Build history of the part. All positions in model axes, mm. A direction names the side the tool comes from. Give positions to 0.01 mm unless a question says otherwise; leave off trailing zeros. Loops run counter-clockwise (first coordinate to the right, second up) from the corner with the lowest first, then second, coordinate; pieces in that order, holes last. Notation, with made-up numbers: (39.25, 15.5) -> (95.25, 15.5) arc R28 cw to (95.25, 46.5) -> close; hole circle Ø4 at (68, 40.5). An arc over 180 degrees is marked (long way). Answer as a JSON object with one key per item and string values. Group by question number.
from build123d import *

# Parameters (mm, degrees)
BOSS_EXTRUDE1_DEPTH = 3
BOSS_EXTRUDE2_DEPTH = 3


with BuildPart() as part:
    # Sketch1 → Boss-Extrude1 (new body)
    with BuildSketch(Plane.XY):
        Polygon((3, -5), (12.522083602, -5), (38.000000001, 65), (38.000000001, 70), (41, 70), (41, 89.999999997), (38.000000001, 89.999999997), (38.000000001, 94.999999997), (28.477916397, 94.999999997), (18.390906449, 67.286167933), (15.571828589, 68.312228362), (8.731425723, 49.518375949), (11.550503583, 48.49231552), (3, 25), (3, 20), (0, 20), (0, 0), (3, 0), align=None)
    extrude(amount=BOSS_EXTRUDE1_DEPTH)

    # Sketch2 → Boss-Extrude2 (add)
    with BuildSketch(Plane(origin=(0, 0, 0), x_dir=(-1, 0, 0), z_dir=(0, 0, -1))):
        Polygon((-7.955671859, 64.929836131), (-3.093269996, 51.57049681), (-8.731425723, 49.518375949), (-15.571828589, 68.312228362), (-18.390906449, 67.286167933), (-28.477916397, 94.999999997), (-18.900316445, 94.999999997), (-14.796074725, 83.723688547), (-11.976996863, 84.749748977), (-5.136593996, 65.955896561), align=None)
    extrude(amount=-BOSS_EXTRUDE2_DEPTH)


solid = part.part
(1) Saw through at C-C on y = 4.5. List the corners of the cut face in (x, z).
(2) Pin check, flat tips, straight feed: pin 1 (1.5 mm diameter, centred on y = 92, z = 1, fed in from +X); pin 2 (1.5 mm diameter, centred on y = 23, z = 1.5, fed in from -X). Stop position of each tip, or through.
(3) Pull direction Y, two halves, no side cores. Call faces 1 (the flat face through (5.559, 58.344, 1.479)), 2 (the flat face through (41, 80, 1)), 3 (the flat face through (13.41, 84.23, 1.48)): pulls with the +Y half, pulls with the -Y half, needs draft (parallel to the pull), parting line crosses it, or undercut.
(4) Saw through at A-A on z = 1. List the corners of the cut face in (x, y).
(5) 3-axis set-ups, long thin cutter, end or side, ignore diameter. For faces 4 (the flat face through (7.335, 36.911, 1.479)), 5 (the flat face through (3, 23, 1)), 6 (the flat face through (38, 92, 1)), 7 (the flat face through (38, 67, 1)): which of +Z, -Z, +X, -X, +Y, -Y reach the whole face in a straight line?
(6) Saw through at B-B on x = 17. List the corners of the cut face in (y, z), plus the area to 3 significant figures.
(7) Probe line 1 along Y through (x, z) = (2, 0.75); line 2 along Y through (x, z) = (12, 1); line 3 along X through (y, z) = (83, 2.15). List the from-to ranges inside material, lowest first. Write a range as [from, to].
Calculated:
{
 "1": {"outline": "(0, 0) -> (15.98, 0) -> (15.98, 3) -> (0, 3) -> close"},
 "2": {"pin 1": "stops at x = 38", "pin 2": "stops at x = 3"},
 "3": {"face 1": "undercut", "face 2": "needs draft", "face 3": "pulls with the +Y half"},
 "4": {"outline": "(0, 0) -> (3, 0) -> (3, -5) -> (12.52, -5) -> (38, 65) -> (38, 70) -> (41, 70) -> (41, 90) -> (38, 90) -> (38, 95) -> (18.9, 95) -> (14.8, 83.72) -> (11.98, 84.75) -> (5.14, 65.96) -> (7.96, 64.93) -> (3.09, 51.57) -> (11.55, 48.49) -> (3, 25) -> (3, 20) -> (0, 20) -> close"},
 "5": {"face 4": "+Z, -Z, -X", "face 5": "+Z, -Z, -X, +Y", "face 6": "+Z, -Z, +X, +Y", "face 7": "+Z, -Z, +X, -Y"},
 "6": {"outline": "(7.3, 0) -> (89.78, 0) -> (89.78, 3) -> (7.3, 3) -> close", "area": "247 mm^2"},
 "7": {"line 1": "y = [0, 20]", "line 2": "y = [-5, 84.74]", "line 3": "x = [11.34, 41]"}
}
